Geometry: final body of the model. Coordinates: model frame, mm. Coordinates: 2 decimals unless noted, no trailing zeros. Loops run counter-clockwise (first coordinate to the right, second up) from the corner with the lowest first, then second, coordinate; pieces in that order, holes last. Notation, with made-up numbers: (40, -27.5) -> (59, -27.5) arc R8 cw to (59, -22.5) -> close; hole circle Ø6 at (65, 35.5). An arc over 180 degrees is marked (long way). One line per item, written item: value. Start each with the question number.
Item 1: Section query A-A on z = 10.5. Return loops of the section in (x, y).
Item 2: Section query C-C on y = 1.15. Give the number of separate pieces and of enclosed holes in the cut face, then the cut area to 3 significant figures.
Item 3: Ray query, probe 1 along Z at (x, y) = (31.75, 1.6); probe 2 along Z at (x, y) = (20, 2.9); probe 3 along X at (y, z) = (0.85, -20.5). Return the intervals inside material, ascending. Write a range as from..to.
Item 4: Section query D-D on z = -21.5. Return loops of the section in (x, y), then the cut area to 3 significant figures.
Item 5: Section query B-B on x = 0. Return loops of the section in (y, z), then the cut area to 3 significant figures.
from build123d import *

# Parameters (mm, degrees)
SKETCH_3_W          = 80
SKETCH_3_H          = 56
EXTRUDE_1_DEPTH     = 5
SKETCH_1_R          = 2.6
SKETCH_1_W          = 40.4
SKETCH_1_H          = 5
CUT_EXTRUDE_1_DEPTH = 5
FILLET_2_R          = 4


with BuildPart() as part:
    # 草图3 → 凸台-拉伸1 (new body)
    with BuildSketch(Plane(origin=(0, 0, 0), x_dir=(1, 0, 0), z_dir=(0, 1, 0))):
        Rectangle(SKETCH_3_W, SKETCH_3_H)
    extrude(amount=EXTRUDE_1_DEPTH)

    # 草图1 → 切除-拉伸1 (cut)
    with BuildSketch(Plane(origin=(0, 0, 0), x_dir=(1, 0, 0), z_dir=(0, 1, 0))):
        with Locations(Location((-31.75, 20.6375, 0), (0, 0, 90))):
            Circle(SKETCH_1_R)
        with Locations(Location((31.75, 20.6375, 0), (0, 0, 90))):
            Circle(SKETCH_1_R)
        with Locations(Location((31.75, -20.6375, 0), (0, 0, 90))):
            Circle(SKETCH_1_R)
        with Locations(Location((-31.75, -20.6375, 0), (0, 0, 90))):
            Circle(SKETCH_1_R)
        with Locations(Location((-22.225, 20.6375, 0), (0, 0, 90))):
            Circle(SKETCH_1_R)
        with Locations(Location((-22.225, -20.6375, 0), (0, 0, 90))):
            Circle(SKETCH_1_R)
        with Locations((0, -10)):
            Rectangle(SKETCH_1_W, SKETCH_1_H)
        with Locations((0, 10)):
            Rectangle(SKETCH_1_W, SKETCH_1_H)
    extrude(amount=CUT_EXTRUDE_1_DEPTH, mode=Mode.SUBTRACT)

    # 圆角2
    fillet_2_edges = [part.edges().sort_by_distance(p)[0] for p in [
        (40, 2.5, 28),
        (-40, 2.5, 28),
        (-40, 2.5, -28),
        (40, 2.5, -28),
    ]]
    fillet(fillet_2_edges, radius=FILLET_2_R)


solid = part.part
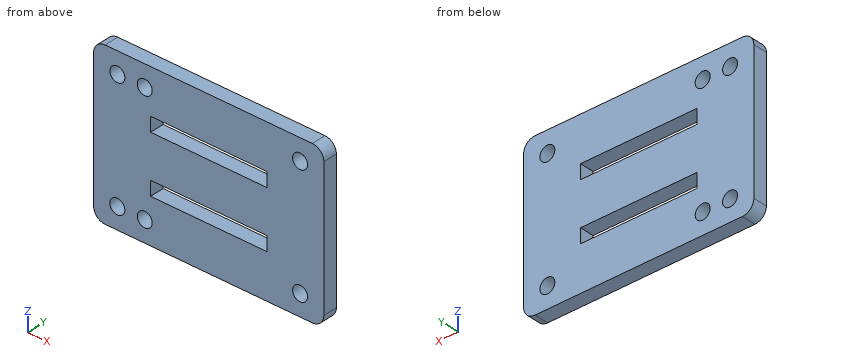
Reply:
1. outline: (-40, 0) -> (-20.2, 0) -> (-20.2, 5) -> (-40, 5) -> close; (20.2, 0) -> (40, 0) -> (40, 5) -> (20.2, 5) -> close
2. separate pieces: 1
2. enclosed holes: 8
2. area: 3,930 mm²
3. probe 1: z = -28..-23.24, -18.04..18.04, 23.24..28
3. probe 2: z = -28..-12.5, -7.5..7.5, 12.5..28
3. probe 3: x = -40..-34.35, -29.15..-24.82, -19.63..29.15, 34.35..40
4. outline: (-40, 0) -> (-34.2, 0) -> (-34.2, 5) -> (-40, 5) -> close; (-29.3, 0) -> (-24.68, 0) -> (-24.68, 5) -> (-29.3, 5) -> close; (-19.77, 0) -> (29.3, 0) -> (29.3, 5) -> (-19.77, 5) -> close; (34.2, 0) -> (40, 0) -> (40, 5) -> (34.2, 5) -> close
4. area: 326 mm²
5. outline: (0, -28) -> (5, -28) -> (5, -12.5) -> (0, -12.5) -> close; (0, -7.5) -> (5, -7.5) -> (5, 7.5) -> (0, 7.5) -> close; (0, 12.5) -> (5, 12.5) -> (5, 28) -> (0, 28) -> close
5. area: 230 mm²
